The listing builds one solid part. Answer for the finished solid, in the listing's coordinates (mm). Coordinates: 2 decimals unless noted, no trailing zeros. Order: outer loops, then holes, each group sorted by start corner. A loop starts at its lowest first (then second) coordinate and runs counter-clockwise, first axis right, second up. Notation, with made-up numbers: M 20.25,63.5 L 30.25,63.5 A19 ccw 30.25,84.5 Z; hole C 54.5,-33 d10. An arc over 180 degrees is marked long. One line per item, written item: value. Start each with the question number.
Q1. The part is cut by section A-A on x = 0. Give the vertices of the cut face in (y, z).
Q2. Straight lines are drawn through the part: line 1 along X through (y, z) = (2.9, 0); line 2 along Z through (x, y) = (1.5, 4.4); line 3 along Z through (x, y) = (72.5, 3.65). For each, find the intervals that lie inside material, in ascending order. Write a range as [from, to].
Q3. The part is cut by section C-C on z = 105. Give the vertices of the cut face in (x, y), then the cut area to 3 significant figures.
Q4. Determine the mould class of faces 1 (the flat face through (2, 0, -2)), 2 (the cylindrical face through (1.08, 2.53, 109.88)), 3 (the cylindrical face through (72.334, 2.535, 78.866)), 4 (the cylindrical face through (5.276, 2.465, -119.884)) for opening direction X: pulls with the +X half, pulls with the -X half, needs draft (parallel to the pull), parting line crosses it, or undercut.
Q5. Each of these flat-tipped pins is pushed along its axis until it touches: pin 1 Ø1 at (x, y) = (77.5, 3.5) entering from -Z; pin 2 Ø2 at (y, z) = (3, 10) entering from +X. Where does it stop, or does it pass through?
Q6. The part is cut by section D-D on x = 105. Give the vertices of the cut face in (y, z), then the cut area to 3 significant figures.
Q7. The part is cut by section B-B on y = 1.45. Give the number of separate pieces and of enclosed holes in the cut face, then the cut area to 3 significant figures.
```python
from build123d import *

# Parameters (mm, degrees)
SKETCH_9_R               = 120
EXTRUDE_1_DEPTH          = 5
PATTERN_CIRCULAR_1_COUNT = 8


with BuildPart() as part:
    # Sketch 9 → Extrude 1 (new body)
    with BuildSketch(Plane(origin=(0, 0, 0), x_dir=(1, 0, 0), z_dir=(0, 1, 0))):
        with Locations(Location((0, 0, 0), (0, 0, 270))):
            Circle(SKETCH_9_R)
    extrude(amount=EXTRUDE_1_DEPTH)

    # Sketch 13 → Hole Wizard 10.0 _10_1 (revolve, cut)
    with BuildSketch(Plane(origin=(105, 5, 0), x_dir=(0, 0, 1), z_dir=(1, 0, 0))):
        Polygon((0, 0), (0, 18.004303095), (5, 15), (5, 0), align=None)
    hole_wizard_10_0_10_1 = revolve(axis=Axis((105, 11.35, 0), (0, -1, 0)), mode=Mode.SUBTRACT)

    # Pattern Circular 1: Hole Wizard 10.0 _10_1 ×8 about axis
    pattern_circular_1_axis = Axis((0, 0, 0), (0, 1, 0))
    for i in range(1, PATTERN_CIRCULAR_1_COUNT):
        add(hole_wizard_10_0_10_1.rotate(pattern_circular_1_axis, i * 360 / PATTERN_CIRCULAR_1_COUNT), mode=Mode.SUBTRACT)


solid = part.part
```
Output:
1. outline: M 0,-120 L 5,-120 L 5,-110 L 0,-110 Z; M 0,-100 L 5,-100 L 5,100 L 0,100 Z; M 0,110 L 5,110 L 5,120 L 0,120 Z
2. line 1: x = [-120, -110], [-100, 100], [110, 120]
2. line 2: z = [-119.99, -109.77], [-100.23, 100.23], [109.77, 119.99]
2. line 3: z = [-95.62, -78.93], [-69.56, 69.56], [78.93, 95.62]
3. outline: M -58.09,0 L -5,0 L -5,5 L -58.09,5 Z; M 5,0 L 58.09,0 L 58.09,5 L 5,5 Z
3. area: 531 mm^2
4. face 1: needs draft
4. face 2: undercut
4. face 3: undercut
4. face 4: parting line crosses it
5. pin 1: stops at z = -92.04
5. pin 2: stops at x = 119.66
6. outline: M 0,-58.09 L 5,-58.09 L 5,-5 L 0,-5 Z; M 0,5 L 5,5 L 5,58.09 L 0,58.09 Z
6. area: 531 mm^2
7. separate pieces: 1
7. enclosed holes: 8
7. area: 44,600 mm^2
